Work out the finished part from the listing and answer in its coordinate system (mm). Face numbers are marked on the shaded views. Round coordinates to 2 decimals unless told otherwise and drop trailing zeros. Loops run counter-clockwise (first coordinate to the right, second up) from the corner with the lowest first, then second, coordinate; pieces in that order, holes last. Notation, with made-up numbers: (37, -5) - (87, -5) arc R25 ccw to (87, 8) - close; hole circle Ø9 at (60.5, -36). An arc over 180 degrees is marked (long way). Return JSON: item names as keys, results as strings.
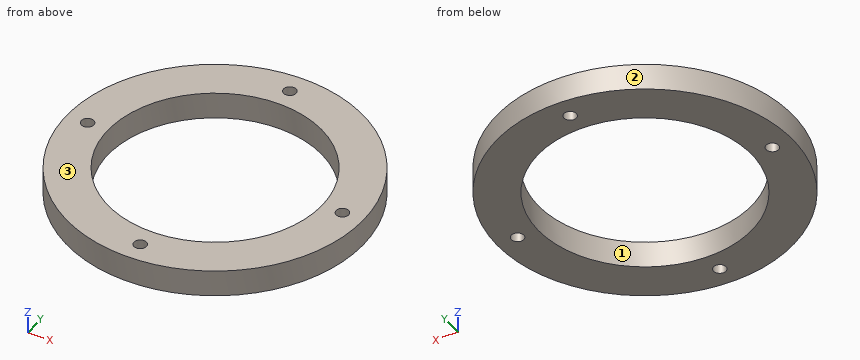
from build123d import *

# Parameters (mm, degrees)
SKETCH1_R           = 35.399999939
BOSS_EXTRUDE1_DEPTH = 6.35
SKETCH2_R           = 25.527
CUT_EXTRUDE1_DEPTH  = 6.35
SKETCH5_R           = 1.5
CUT_EXTRUDE2_DEPTH  = 6.35


with BuildPart() as part:
    # Sketch1 → Boss-Extrude1 (new body)
    with BuildSketch(Plane.XY):
        Circle(SKETCH1_R)
    extrude(amount=BOSS_EXTRUDE1_DEPTH)

    # Sketch2 → Cut-Extrude1 (cut)
    with BuildSketch(Plane.XY.offset(6.35)):
        Circle(SKETCH2_R)
    extrude(amount=-CUT_EXTRUDE1_DEPTH, mode=Mode.SUBTRACT)

    # Sketch5 → Cut-Extrude2 (cut)
    with BuildSketch(Plane.XY.offset(6.35)):
        with Locations((0, 30.400000033)):
            Circle(SKETCH5_R)
        with Locations((30.400000033, 0)):
            Circle(SKETCH5_R)
        with Locations((0, -30.400000033)):
            Circle(SKETCH5_R)
        with Locations((-30.400000033, 0)):
            Circle(SKETCH5_R)
    extrude(amount=-CUT_EXTRUDE2_DEPTH, mode=Mode.SUBTRACT)


solid = part.part
1) Section A-A (y = 0) is taken. Give the vertices of the cut face in (x, z).
Verdict:
{"outline": "(-35.4, 0) - (-31.9, 0) - (-31.9, 6.35) - (-35.4, 6.35) - close; (-28.9, 0) - (-25.53, 0) - (-25.53, 6.35) - (-28.9, 6.35) - close; (25.53, 0) - (28.9, 0) - (28.9, 6.35) - (25.53, 6.35) - close; (31.9, 0) - (35.4, 0) - (35.4, 6.35) - (31.9, 6.35) - close"}
2) Determine the mould class of the marked faces 1, 2 and 3 for opening direction Y: pulls with the +Y half, pulls with the -Y half, needs draft (parallel to the pull), parting line crosses it, or undercut.
Verdict:
{"face 1": "undercut", "face 2": "parting line crosses it", "face 3": "needs draft"}
3) Section D-D (z = 5) is taken. Give the vertices of the cut face in (x, y), and give its area (3 significant figures).
Verdict:
{"outline": "circle Ø70.8 at (0, 0); hole circle Ø3 at (-30.4, 0); hole circle Ø51.05 at (0, 0); hole circle Ø3 at (0, -30.4); hole circle Ø3 at (0, 30.4); hole circle Ø3 at (30.4, 0)", "area": "1,860 mm2"}
4) Flat-ended cylindrical pins translate along their axes: pin 1 (1.5 mm diameter, centred on x = -19.5, z = 2.5, fed in from -Y); pin 2 (1 mm diameter, centred on x = 22.5, z = 5, fed in from -Y); pin 3 (2 mm diameter, centred on y = 25.5, z = 1.5, fed in from -X). Find the tip coordinate at first contact, or state that the pin passes through.
Verdict:
{"pin 1": "stops at y = -30.03", "pin 2": "stops at y = -27.73", "pin 3": "stops at x = -25.55"}
5) Section B-B (x = 9.5) is taken. Give the vertices of the cut face in (y, z).
Verdict:
{"outline": "(-34.1, 0) - (-23.69, 0) - (-23.69, 6.35) - (-34.1, 6.35) - close; (23.69, 0) - (34.1, 0) - (34.1, 6.35) - (23.69, 6.35) - close"}
6) Find the intervals of material crossed by L1, parallel to Y at x = -7.5, z = 2.5; L2, parallel to X at y = -1, z = 0.5; L3, parallel to X at y = -8, z = 5.75, in increasing order.
Verdict:
{"L1": "y = -34.6 to -24.4, 24.4 to 34.6", "L2": "x = -35.39 to -31.52, -29.28 to -25.51, 25.51 to 29.28, 31.52 to 35.39", "L3": "x = -34.48 to -24.24, 24.24 to 34.48"}
7) Section C-C (y = 19.5) is taken. Give the vertices of the cut face in (x, z), and give its area (3 significant figures).
Verdict:
{"outline": "(-29.55, 0) - (-16.47, 0) - (-16.47, 6.35) - (-29.55, 6.35) - close; (16.47, 0) - (29.55, 0) - (29.55, 6.35) - (16.47, 6.35) - close", "area": "166 mm2"}
